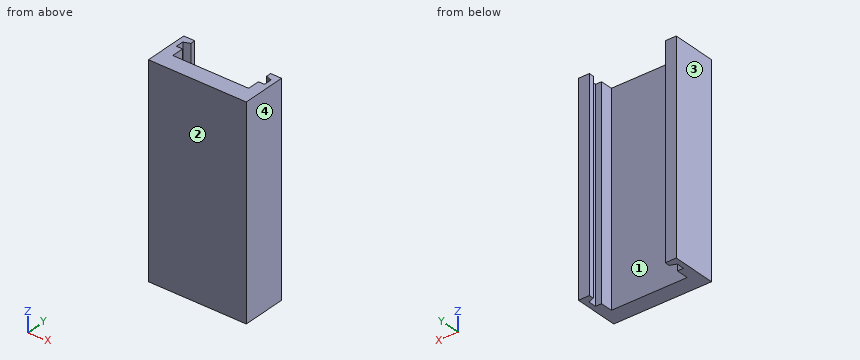
```python
from build123d import *

# Parameters (mm, degrees)
F0_W        = 20
F0_H        = 42
F1_DEPTH    = 9
F2_W        = 15.5
F2_H        = 1.5
F2_H_2      = 1.6
F2_W_2      = 1.25
F2_H_3      = 2.5
F3_DEPTH    = 42.001
F4_T4_DEPTH = 48.7433158126
F5_T4_DEPTH = 49.2642981969


# Not quite as in the source:
# - a fillet or chamfer that OpenCascade refuses, or shapes differently, is made with other operations: its cross-section is extruded or revolved along the edge and cut away or added


with BuildPart() as f1:
    # F0 (on Front) → F1 (new body)
    with BuildSketch(Plane.XZ):
        Rectangle(F0_W, F0_H)
    extrude(amount=F1_DEPTH)

    # F2 (on face) → F3 (cut, through all)
    with BuildSketch(Plane.XY.offset(21)):
        with Locations((0, -0.75)):
            Rectangle(F2_W, F2_H)
        with Locations((0, -2.3)):
            Rectangle(F2_W, F2_H_2)
        with Locations((-8.375, -2.3)):
            Rectangle(F2_W_2, F2_H_2)
        with Locations((8.375, -2.3)):
            Rectangle(F2_W_2, F2_H_2)
        with Locations((0, -4.35)):
            Rectangle(F2_W, F2_H_3)
    extrude(amount=-F3_DEPTH, mode=Mode.SUBTRACT)

    # F4: chamfer of 1.3 x 0.5 on 1 edges, made by hand


with BuildPart() as f4_tool2:
    # F4_s3 → F4_t4 (new body)
    with BuildSketch(Plane.XY.offset(24.3716579063)):
        Polygon((-7.75, -1), (-9.05, -1.5), (-7.75, -1.5), align=None)
    extrude(amount=-F4_T4_DEPTH)

    split(bisect_by=Plane.YZ.offset(-9), keep=Keep.TOP)


with BuildPart() as f1_1:
    add(f1.part)

    # F4_t1: cut F4_tool2
    add(f4_tool2.part, mode=Mode.SUBTRACT)

    # F5: chamfer of 1.4 x 0.5 on 1 edges, made by hand


with BuildPart() as f5_tool2:
    # F5_s3 → F5_t4 (new body)
    with BuildSketch(Plane.XY.offset(24.6321490984)):
        Polygon((9.15, -1.5), (7.75, -1), (7.75, -1.5), align=None)
    extrude(amount=-F5_T4_DEPTH)

    split(bisect_by=Plane.YZ.offset(9), keep=Keep.BOTTOM)


with BuildPart() as f1_2:
    add(f1_1.part)

    # F5_t1: cut F5_tool2
    add(f5_tool2.part, mode=Mode.SUBTRACT)


solid = f1_2.part
```
CAD build for the part. Positions are in the model's coordinates, mm. Face numbers are marked on the shaded views. Coordinates: 2 decimals unless noted, no trailing zeros. Order: outer loops, then holes, each group sorted by start corner. A loop starts at its lowest first (then second) coordinate and runs counter-clockwise, first axis right, second up. Notation, with made-up numbers: (74, 14.25) -> (107, 14.25) arc R25 ccw to (107, 52.25) -> close; hole circle Ø1 at (4.5, -6). An arc over 180 degrees is marked (long way). Use one line per item in the form item = value. Start each with the question number.
1) Drill centre lines: L1, parallel to X at y = -1.75, z = 19; L2, parallel to X at y = -4, z = -19; L3, parallel to Y at x = 2.25, z = -14.5. Where is each one in solid material? Low to high. Write a range as [from, to].
2) Band-saw the part on C-C on x = 4. Give the cut face in (y, z), then the cut area to 3 significant figures.
3) Band-saw the part on B-B on z = 14.5. Give the cut face in (x, y).
4) Band-saw the part on A-A on y = -5. Give the cut face in (x, z), then the cut area to 3 significant figures.
5) Pull direction X, two halves, no side cores. Call the marked faces 1, 2, 3 and 4: +X half, -X half, draft (parallel to the pull), parting line (faces both ways), or undercut.
Entries:
q1.L1 = [-10, -9], [9, 10]
q1.L2 = [-10, -7.75], [7.75, 10]
q1.L3 = [-9, -5.6]
q2.outline = (-9, -21) -> (-5.6, -21) -> (-5.6, 21) -> (-9, 21) -> close
q2.area = 143 mm2
q3.outline = (-10, -9) -> (10, -9) -> (10, 0) -> (7.75, 0) -> (7.75, -1) -> (9, -1.45) -> (9, -3.1) -> (7.75, -3.1) -> (7.75, -5.6) -> (-7.75, -5.6) -> (-7.75, -3.1) -> (-9, -3.1) -> (-9, -1.48) -> (-7.75, -1) -> (-7.75, 0) -> (-10, 0) -> close
q4.outline = (-10, -21) -> (-7.75, -21) -> (-7.75, 21) -> (-10, 21) -> close; (7.75, -21) -> (10, -21) -> (10, 21) -> (7.75, 21) -> close
q4.area = 189 mm2
q5.face_1 = undercut
q5.face_2 = draft
q5.face_3 = -X half
q5.face_4 = +X half
